from build123d import *

# Parameters (mm, degrees)
DECK_DEPTH                          = 3
CUT_DECKPOSTS_M5_DEPTH              = 207.177108332
CUT_DECKPOSTS_M5_DEPTH_BACK         = 207.177108332
SK_DECKPOSTS_M5_R                   = 2.75
CUT_LIDARMOUNT_DEPTH                = 207.177108332
CUT_LIDARMOUNT_DEPTH_BACK           = 207.177108332
SK_LIDARMOUNT_R                     = 1.7
SK_LIDARMOUNT_R_2                   = 10
CUT_PI5_M2P5_DEPTH                  = 207.177108332
CUT_PI5_M2P5_DEPTH_BACK             = 207.177108332
SK_PI5_M2P5_R                       = 1.35
CUT_DECKGRID_M3_DEPTH               = 207.177108332
CUT_DECKGRID_M3_DEPTH_BACK          = 207.177108332
SK_DECKGRID_M3_R                    = 1.7
CUT_ESTOP_22MM_DEPTH                = 207.177108332
CUT_ESTOP_22MM_DEPTH_BACK           = 207.177108332
SK_ESTOP_22MM_R                     = 11.25
CUT_CAMERAMOUNT_M4_DEPTH            = 207.177108332
CUT_CAMERAMOUNT_M4_DEPTH_BACK       = 207.177108332
SK_CAMERAMOUNT_M4_R                 = 2.25
CUT_INDICATORLIGHTS_16MM_DEPTH      = 207.177108332
CUT_INDICATORLIGHTS_16MM_DEPTH_BACK = 207.177108332
SK_INDICATORLIGHTS_R                = 8
CUT_DECKPASSTHRU_DEPTH              = 207.177108332
CUT_DECKPASSTHRU_DEPTH_BACK         = 207.177108332


with BuildPart() as part:
    # SK_Deck → Deck (new body)
    with BuildSketch(Plane(origin=(0, 0, 0), x_dir=(1, 0, 0), z_dir=(0, 1, 0))):
        with BuildLine():
            Line((160, -110), (160, 110))
            ThreePointArc((160, 110), (154.142135624, 124.142135624), (140, 130))
            Line((140, 130), (-140, 130))
            ThreePointArc((-140, 130), (-154.142135624, 124.142135624), (-160, 110))
            Line((-160, 110), (-160, -110))
            ThreePointArc((-160, -110), (-154.142135624, -124.142135624), (-140, -130))
            Line((-140, -130), (140, -130))
            ThreePointArc((140, -130), (154.142135624, -124.142135624), (160, -110))
        make_face()
    extrude(amount=DECK_DEPTH)

    # SK_DeckPosts_M5 → Cut_DeckPosts_M5 (cut, two sides: drawn at the far end of the back side and taken through both)
    with BuildSketch(Plane(origin=(0, 0, 0), x_dir=(1, 0, 0), z_dir=(0, 1, 0)).offset(-CUT_DECKPOSTS_M5_DEPTH_BACK)):
        with Locations(Location((140, 110, 0), (0, 0, 270))):
            Circle(SK_DECKPOSTS_M5_R)
        with Locations(Location((140, -110, 0), (0, 0, 270))):
            Circle(SK_DECKPOSTS_M5_R)
        with Locations(Location((-140, 110, 0), (0, 0, 270))):
            Circle(SK_DECKPOSTS_M5_R)
        with Locations(Location((-140, -110, 0), (0, 0, 270))):
            Circle(SK_DECKPOSTS_M5_R)
    extrude(amount=CUT_DECKPOSTS_M5_DEPTH + CUT_DECKPOSTS_M5_DEPTH_BACK, mode=Mode.SUBTRACT)

    # SK_LidarMount → Cut_LidarMount (cut, two sides: drawn at the far end of the back side and taken through both)
    with BuildSketch(Plane(origin=(0, 0, 0), x_dir=(1, 0, 0), z_dir=(0, 1, 0)).offset(-CUT_LIDARMOUNT_DEPTH_BACK)):
        with Locations(Location((20, 20, 0), (0, 0, 270))):
            Circle(SK_LIDARMOUNT_R)
        with Locations(Location((20, -20, 0), (0, 0, 270))):
            Circle(SK_LIDARMOUNT_R)
        with Locations(Location((-20, 20, 0), (0, 0, 270))):
            Circle(SK_LIDARMOUNT_R)
        with Locations(Location((-20, -20, 0), (0, 0, 270))):
            Circle(SK_LIDARMOUNT_R)
        with Locations(Location((0, 0, 0), (0, 0, 270))):
            Circle(SK_LIDARMOUNT_R_2)
    extrude(amount=CUT_LIDARMOUNT_DEPTH + CUT_LIDARMOUNT_DEPTH_BACK, mode=Mode.SUBTRACT)

    # SK_Pi5_M2p5 → Cut_Pi5_M2p5 (cut, two sides: drawn at the far end of the back side and taken through both)
    with BuildSketch(Plane(origin=(0, 0, 0), x_dir=(1, 0, 0), z_dir=(0, 1, 0)).offset(-CUT_PI5_M2P5_DEPTH_BACK)):
        with Locations(Location((-119, 40.5, 0), (0, 0, 270))):
            Circle(SK_PI5_M2P5_R)
        with Locations(Location((-119, 89.5, 0), (0, 0, 270))):
            Circle(SK_PI5_M2P5_R)
        with Locations(Location((-61, 40.5, 0), (0, 0, 270))):
            Circle(SK_PI5_M2P5_R)
        with Locations(Location((-61, 89.5, 0), (0, 0, 270))):
            Circle(SK_PI5_M2P5_R)
    extrude(amount=CUT_PI5_M2P5_DEPTH + CUT_PI5_M2P5_DEPTH_BACK, mode=Mode.SUBTRACT)

    # SK_DeckGrid_M3 → Cut_DeckGrid_M3 (cut, two sides: drawn at the far end of the back side and taken through both)
    with BuildSketch(Plane(origin=(0, 0, 0), x_dir=(1, 0, 0), z_dir=(0, 1, 0)).offset(-CUT_DECKGRID_M3_DEPTH_BACK)):
        with Locations(Location((-120, -40, 0), (0, 0, 270))):
            Circle(SK_DECKGRID_M3_R)
        with Locations(Location((-120, -60, 0), (0, 0, 270))):
            Circle(SK_DECKGRID_M3_R)
        with Locations(Location((-120, -80, 0), (0, 0, 270))):
            Circle(SK_DECKGRID_M3_R)
        with Locations(Location((-120, -100, 0), (0, 0, 270))):
            Circle(SK_DECKGRID_M3_R)
        with Locations(Location((-100, -40, 0), (0, 0, 270))):
            Circle(SK_DECKGRID_M3_R)
        with Locations(Location((-100, -60, 0), (0, 0, 270))):
            Circle(SK_DECKGRID_M3_R)
        with Locations(Location((-100, -80, 0), (0, 0, 270))):
            Circle(SK_DECKGRID_M3_R)
        with Locations(Location((-100, -100, 0), (0, 0, 270))):
            Circle(SK_DECKGRID_M3_R)
        with Locations(Location((-80, -40, 0), (0, 0, 270))):
            Circle(SK_DECKGRID_M3_R)
        with Locations(Location((-80, -60, 0), (0, 0, 270))):
            Circle(SK_DECKGRID_M3_R)
        with Locations(Location((-80, -80, 0), (0, 0, 270))):
            Circle(SK_DECKGRID_M3_R)
        with Locations(Location((-80, -100, 0), (0, 0, 270))):
            Circle(SK_DECKGRID_M3_R)
        with Locations(Location((-60, -40, 0), (0, 0, 270))):
            Circle(SK_DECKGRID_M3_R)
        with Locations(Location((-60, -60, 0), (0, 0, 270))):
            Circle(SK_DECKGRID_M3_R)
        with Locations(Location((-60, -80, 0), (0, 0, 270))):
            Circle(SK_DECKGRID_M3_R)
        with Locations(Location((-60, -100, 0), (0, 0, 270))):
            Circle(SK_DECKGRID_M3_R)
        with Locations(Location((-40, -40, 0), (0, 0, 270))):
            Circle(SK_DECKGRID_M3_R)
        with Locations(Location((-40, -60, 0), (0, 0, 270))):
            Circle(SK_DECKGRID_M3_R)
        with Locations(Location((-40, -80, 0), (0, 0, 270))):
            Circle(SK_DECKGRID_M3_R)
        with Locations(Location((-40, -100, 0), (0, 0, 270))):
            Circle(SK_DECKGRID_M3_R)
    extrude(amount=CUT_DECKGRID_M3_DEPTH + CUT_DECKGRID_M3_DEPTH_BACK, mode=Mode.SUBTRACT)

    # SK_EStop_22mm → Cut_EStop_22mm (cut, two sides: drawn at the far end of the back side and taken through both)
    with BuildSketch(Plane(origin=(0, 0, 0), x_dir=(1, 0, 0), z_dir=(0, 1, 0)).offset(-CUT_ESTOP_22MM_DEPTH_BACK)):
        with Locations(Location((-130, 0, 0), (0, 0, 270))):
            Circle(SK_ESTOP_22MM_R)
    extrude(amount=CUT_ESTOP_22MM_DEPTH + CUT_ESTOP_22MM_DEPTH_BACK, mode=Mode.SUBTRACT)

    # SK_CameraMount_M4 → Cut_CameraMount_M4 (cut, two sides: drawn at the far end of the back side and taken through both)
    with BuildSketch(Plane(origin=(0, 0, 0), x_dir=(1, 0, 0), z_dir=(0, 1, 0)).offset(-CUT_CAMERAMOUNT_M4_DEPTH_BACK)):
        with Locations(Location((120, 30, 0), (0, 0, 270))):
            Circle(SK_CAMERAMOUNT_M4_R)
        with Locations(Location((120, -30, 0), (0, 0, 270))):
            Circle(SK_CAMERAMOUNT_M4_R)
        with Locations(Location((140, 30, 0), (0, 0, 270))):
            Circle(SK_CAMERAMOUNT_M4_R)
        with Locations(Location((140, -30, 0), (0, 0, 270))):
            Circle(SK_CAMERAMOUNT_M4_R)
    extrude(amount=CUT_CAMERAMOUNT_M4_DEPTH + CUT_CAMERAMOUNT_M4_DEPTH_BACK, mode=Mode.SUBTRACT)

    # SK_IndicatorLights → Cut_IndicatorLights_16mm (cut, two sides: drawn at the far end of the back side and taken through both)
    with BuildSketch(Plane(origin=(0, 0, 0), x_dir=(1, 0, 0), z_dir=(0, 1, 0)).offset(-CUT_INDICATORLIGHTS_16MM_DEPTH_BACK)):
        with Locations(Location((130, 75, 0), (0, 0, 270))):
            Circle(SK_INDICATORLIGHTS_R)
        with Locations(Location((130, -75, 0), (0, 0, 270))):
            Circle(SK_INDICATORLIGHTS_R)
    extrude(amount=CUT_INDICATORLIGHTS_16MM_DEPTH + CUT_INDICATORLIGHTS_16MM_DEPTH_BACK, mode=Mode.SUBTRACT)

    # SK_DeckPassThru → Cut_DeckPassThru (cut, two sides: drawn at the far end of the back side and taken through both)
    with BuildSketch(Plane(origin=(0, 0, 0), x_dir=(1, 0, 0), z_dir=(0, 1, 0)).offset(-CUT_DECKPASSTHRU_DEPTH_BACK)):
        with BuildLine():
            Line((-10, 66), (30, 66))
            ThreePointArc((30, 66), (36, 60), (30, 54))
            Line((30, 54), (-10, 54))
            ThreePointArc((-10, 54), (-16, 60), (-10, 66))
        make_face()
        with BuildLine():
            Line((-10, -54), (30, -54))
            ThreePointArc((30, -54), (36, -60), (30, -66))
            Line((30, -66), (-10, -66))
            ThreePointArc((-10, -66), (-16, -60), (-10, -54))
        make_face()
    extrude(amount=CUT_DECKPASSTHRU_DEPTH + CUT_DECKPASSTHRU_DEPTH_BACK, mode=Mode.SUBTRACT)


solid = part.part
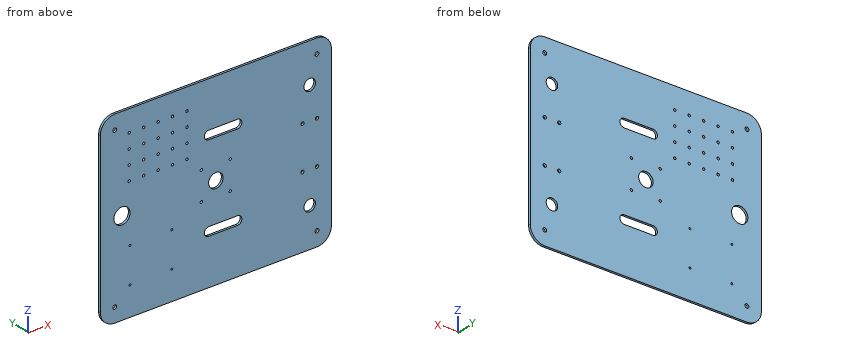
For this review, take the finished solid that the model builds, in its own axes (mm). Round coordinates to 2 decimals unless told otherwise and drop trailing zeros. Loops run counter-clockwise (first coordinate to the right, second up) from the corner with the lowest first, then second, coordinate; pieces in that order, holes last. Notation, with made-up numbers: (4, 35.25) - (25, 35.25) arc R19 ccw to (25, 61.25) - close; hole circle Ø8 at (79, 35.5). An arc over 180 degrees is marked (long way). One line per item, written item: value. Start each with the question number.
Item 1: For L1, parallel to Z at x = -20, y = 1.9; L2, parallel to Z at x = -79.5, y = 2.15; L3, parallel to Z at x = -100, y = 0.7, list the stretches that pass through material, from the lowest coordinate up.
Item 2: Take a section at C-C (y = 1.8). State how many separate pieces and enclosed holes the cut face has, plus the area to 3 significant figures.
Item 3: Take a section at B-B (x = 130). Give the boundary of the cut face in (y, z).
Item 4: Take a section at A-A (z = 0). Give the boundary of the cut face in (x, y), plus the area to 4 significant figures.
Answer below:
1. L1: z = -130 to -21.7, -18.3 to 18.3, 21.7 to 130
1. L2: z = -130 to 38.38, 41.62 to 58.38, 61.62 to 78.38, 81.62 to 98.38, 101.62 to 130
1. L3: z = -130 to 38.3, 41.7 to 58.3, 61.7 to 78.3, 81.7 to 98.3, 101.7 to 130
2. separate pieces: 1
2. enclosed holes: 42
2. area: 80,200 mm2
3. outline: (0, -130) - (3, -130) - (3, -83) - (0, -83) - close; (0, -67) - (3, -67) - (3, 67) - (0, 67) - close; (0, 83) - (3, 83) - (3, 130) - (0, 130) - close
4. outline: (-160, 0) - (-141.25, 0) - (-141.25, 3) - (-160, 3) - close; (-118.75, 0) - (-10, 0) - (-10, 3) - (-118.75, 3) - close; (10, 0) - (160, 0) - (160, 3) - (10, 3) - close
4. area: 832.5 mm2
